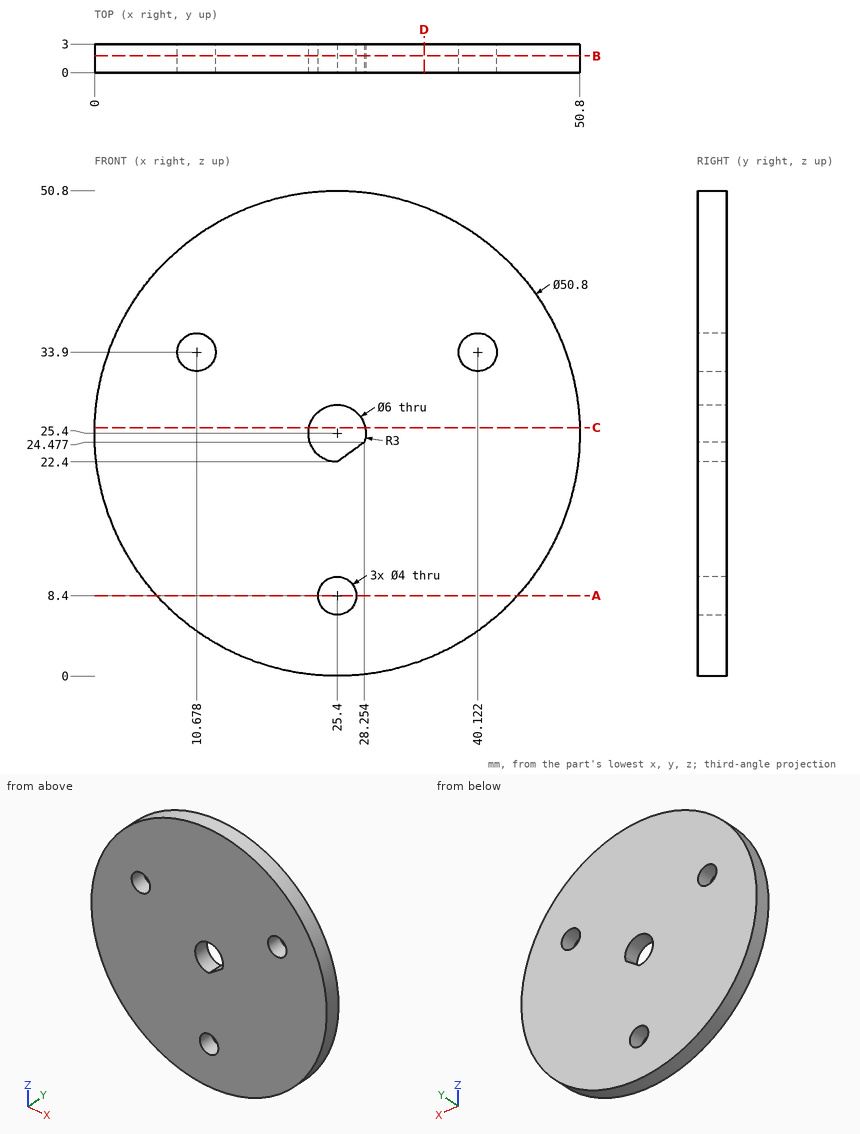
Answer from the drawing. Dimensions are ordinates in mm from the lowest x, y and z of the part. Coordinates: 2 decimals unless noted, no trailing zeros. Order: outer loops, then holes, each group sorted by start corner. A loop starts at its lowest first (then second) coordinate and runs counter-clockwise, first axis right, second up. Notation, with made-up numbers: (78, 81) - (132, 81) arc R21 ccw to (132, 91) - close; hole circle Ø1 at (8.5, 1.25). An arc over 180 degrees is marked (long way). Put each result on its own line as item: value. Start each with the question number.
1) Find section A-A (z = 8.4). Give the vertices of the cut face in (x, y).
2) Flat-ended cylindrical pins translate along their axes: pin 1 (1.5 mm diameter, centred on x = 14.5, y = 2, fed in from -Z); pin 2 (3.5 mm diameter, centred on x = 10.68, z = 33.9, fed in from +Y); pin 3 (1 mm diameter, centred on y = 1.5, z = 22.5, fed in from +X). Find the tip coordinate at first contact, or state that the pin passes through.
3) Find section B-B (y = 1.75). Give the vertices of the cut face in (x, z) (1 decimal).
4) Find section C-C (z = 26). Give the vertices of the cut face in (x, y).
5) Find section D-D (x = 34.5). Give the vertices of the cut face in (y, z).
6) Find the intervals of material crossed by line 1 (X direction, y = 2.5, z = 25.5); line 2 (X direction, y = 2.15, z = 33.9) (1 decimal); line 3 (X direction, y = 2.65, z = 33.5) (1 decimal), in increasing order. Write a range as from..to.
Results list:
1. outline: (6.53, 0) - (23.4, 0) - (23.4, 3) - (6.53, 3) - close; (27.4, 0) - (44.27, 0) - (44.27, 3) - (27.4, 3) - close
2. pin 1: stops at z = 2.12
2. pin 2: passes through
2. pin 3: stops at x = 50.69
3. outline: circle Ø50.8 at (25.4, 25.4); hole circle Ø4 at (10.7, 33.9); hole circle Ø4 at (25.4, 8.4); hole (25.4, 22.4) - (28.3, 24.5) arc R3 ccw (long way) to start; hole circle Ø4 at (40.1, 33.9)
4. outline: (0.01, 0) - (22.46, 0) - (22.46, 3) - (0.01, 3) - close; (28.34, 0) - (50.79, 0) - (50.79, 3) - (28.34, 3) - close
5. outline: (0, 1.69) - (3, 1.69) - (3, 49.11) - (0, 49.11) - close
6. line 1: x = 0..22.4, 28.4..50.8
6. line 2: x = 1.5..8.7, 12.7..38.1, 42.1..49.3
6. line 3: x = 1.3..8.7, 12.6..38.2, 42.1..49.5
